Here's how the part is built. I have some questions about the finished solid (model axes, mm). Face numbers are marked on the shaded views. A direction names the side the tool comes from. Coordinates: 2 decimals unless noted, no trailing zeros. Write each loop counter-clockwise with the first axis right and the second up, starting at its lowest first coordinate (ties: lowest second). Pieces come first, ordered by that corner, then holes.
Item 1: For the marked faces 1 and 2, which set-ups out of +Z, -Z, +X, -X, +Y, -Y let a thin tool reach every point of the face, with its end or its side?
Item 2: If I drill on line 1 (Y direction, x = -54, z = -93.5); line 2 (Z direction, x = -52.5, y = -6); line 3 (Z direction, x = -1, y = -5), over which ranges is the centre line in solid material (lowest first)?
Item 3: I'm going to push flat-ended pins straight in: pin 1 Ø1.5 at (x, y) = (-15, -5) entering from +Z; pin 2 Ø10 at (x, y) = (32, 5.5) entering from -Z; pin 3 Ø8 at (y, z) = (-2, 27.5) entering from -X. Where does each tip first touch, or does it pass through?
Item 4: If we section it at C-C (y = -4): Please give me the cut outline in (x, z).
Item 5: If we section it at D-D (z = -138): Please give me the cut outline in (x, y), then the cut area to 3 significant figures.
Item 6: If we section it at B-B (x = 0): Please give me the cut outline in (y, z), then the cut area to 3 significant figures.
Item 7: If we section it at A-A (z = 0): Please give me the cut outline in (x, y), then the cut area to 3 significant figures.
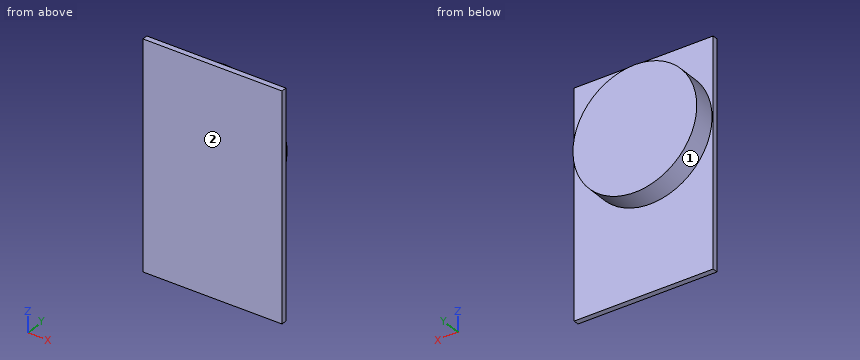
from build123d import *

# Parameters (mm, degrees)
SKETCH1_R           = 71.25
BOSS_EXTRUDE1_DEPTH = 12.6
SKETCH2_W           = 160
SKETCH2_H           = 260
BOSS_EXTRUDE2_DEPTH = 6.35


with BuildPart() as part:
    # Sketch1 → Boss-Extrude1 (new, symmetric)
    with BuildSketch(Plane(origin=(0, 0, 0), x_dir=(1, 0, 0), z_dir=(0, 1, 0))):
        with Locations(Location((0, 0, 0), (0, 0, 270))):
            Circle(SKETCH1_R)
    extrude(amount=BOSS_EXTRUDE1_DEPTH, both=True)

    # Sketch2 → Boss-Extrude2 (add)
    with BuildSketch(Plane.XZ.offset(12.6)):
        with Locations((7.5, -40)):
            Rectangle(SKETCH2_W, SKETCH2_H)
    extrude(amount=BOSS_EXTRUDE2_DEPTH)


solid = part.part
Answer list:
1. face 1: +Y
1. face 2: +Z, -Z, +X, -X, -Y
2. line 1: y = -18.95 to -12.6
2. line 2: z = -48.17 to 48.17
2. line 3: z = -71.24 to 71.24
3. pin 1: stops at z = 69.81
3. pin 2: stops at z = -65.94
3. pin 3: stops at x = -67.26
4. outline: circle Ø142.5 at (0, 0)
5. outline: (-72.5, -18.95) - (87.5, -18.95) - (87.5, -12.6) - (-72.5, -12.6) - close
5. area: 1,020 mm2
6. outline: (-18.95, -170) - (-12.6, -170) - (-12.6, -71.25) - (12.6, -71.25) - (12.6, 71.25) - (-12.6, 71.25) - (-12.6, 90) - (-18.95, 90) - close
6. area: 5,240 mm2
7. outline: (-72.5, -18.95) - (87.5, -18.95) - (87.5, -12.6) - (71.25, -12.6) - (71.25, 12.6) - (-71.25, 12.6) - (-71.25, -12.6) - (-72.5, -12.6) - close
7. area: 4,610 mm2
